```python
from build123d import *

# Parameters (mm, degrees)
BOSS_EXTRUDE1_DEPTH = 10
CUT_EXTRUDE1_DEPTH  = 7
CHAMFER2_SIZE       = 1
CHAMFER3_SIZE       = 1
SKETCH3_R           = 2.5
CUT_EXTRUDE2_DEPTH  = 10
SHELL2_START        = -7
SHELL2_DEPTH        = 14
CHAMFER4_SIZE       = 1


# Read off the part's stored shape, not the designer's step: Shell2
with BuildPart() as part:
    # Sketch1 → Boss-Extrude1 (new, symmetric)
    with BuildSketch(Plane.XY):
        with BuildLine():
            Line((-12.5, 10), (12.5, 10))
            ThreePointArc((12.5, 10), (22.5, 0), (12.5, -10))
            Line((12.5, -10), (-12.5, -10))
            ThreePointArc((-12.5, -10), (-22.5, 0), (-12.5, 10))
        make_face()
    extrude(amount=BOSS_EXTRUDE1_DEPTH, both=True)

    # Sketch2 → Cut-Extrude1 (cut, symmetric)
    with BuildSketch(Plane.XY):
        with BuildLine():
            Line((-12.5, 10), (-2.5, 10))
            Line((-2.5, 10), (-2.5, -10))
            Line((-2.5, -10), (-12.5, -10))
            ThreePointArc((-12.5, -10), (-22.5, 0), (-12.5, 10))
        make_face()
    extrude(amount=CUT_EXTRUDE1_DEPTH, both=True, mode=Mode.SUBTRACT)

    # Chamfer2
    chamfer2_edges = [part.edges().sort_by_distance(p)[0] for p in [
        (-22.5, 0, -7),
        (-7.5, 10, -7),
        (-7.5, -10, -7),
        (-22.5, 0, 7),
        (-7.5, -10, 7),
        (-7.5, 10, 7),
    ]]
    chamfer(chamfer2_edges, length=CHAMFER2_SIZE)

    # Chamfer3
    chamfer3_edges = [part.edges().sort_by_distance(p)[0] for p in [
        (22.5, 0, 10),
        (0, 10, 10),
        (-22.5, 0, 10),
        (0, 10, -10),
        (22.5, 0, -10),
        (0, -10, -10),
        (-22.5, 0, -10),
        (0, -10, 10),
    ]]
    chamfer(chamfer3_edges, length=CHAMFER3_SIZE)

    # Sketch3 → Cut-Extrude2 (cut, symmetric)
    with BuildSketch(Plane.XY):
        with Locations((-12.5, 0)):
            Circle(SKETCH3_R)
    extrude(amount=CUT_EXTRUDE2_DEPTH, both=True, mode=Mode.SUBTRACT)

    # Shell2 outline → Shell2 (cut)
    with BuildSketch(Plane.XY.offset(SHELL2_START)):
        with BuildLine():
            Line((12.5, 7), (-2.5, 7))
            Line((-2.5, 7), (-2.5, -7))
            Line((-2.5, -7), (12.5, -7))
            ThreePointArc((12.5, -7), (19.5, 0), (12.5, 7))
        make_face()
    extrude(amount=SHELL2_DEPTH, mode=Mode.SUBTRACT)

    # Chamfer4
    chamfer4_edges = [part.edges().sort_by_distance(p)[0] for p in [
        (-2.5, -10, 0),
        (-2.5, 10, 0),
    ]]
    chamfer(chamfer4_edges, length=CHAMFER4_SIZE)


solid = part.part
```
Geometry check sheet. Reference: the model listing, model coordinates, mm. A direction names the side the tool comes from. Coordinates: 2 decimals unless noted, no trailing zeros. Write each loop counter-clockwise with the first axis right and the second up, starting at its lowest first coordinate (ties: lowest second). Pieces come first, ordered by that corner, then holes. Notation, with made-up numbers: M 57.5,9.5 L 114.5,9.5 A3 ccw 114.5,14.5 Z; hole C -17.75,-37.75 d7. An arc over 180 degrees is marked long. Use one line per item in the form item = value. Start each with the question number.
1) Release check for a two-part mould opening along Z. For faces 1 (the flat face through (5, 10, 0)), 2 (the cylindrical face through (19.5, -0.15, -0.1)), 3 (the flat face through (0.2, -9.5, 9.5)) record: pulls with the +Z half, pulls with the -Z half, needs draft (parallel to the pull), parting line crosses it, or undercut.
2) Section check A-A on x = -4.5. Enter the section's corners in (y, z).
3) Section check B-B on z = -7.5. Enter the section's corners in (x, y).
4) Section check C-C on y = 0. Enter the section's corners in (x, z), and give its area (3 significant figures).
5) Go/stop test with flat-tipped pins: pin 1 Ø1.5 at (x, z) = (17.5, -6.5) entering from -Y; pin 2 Ø1.6 at (y, z) = (-8.5, -3.5) entering from -X; pin 3 Ø6 at (x, y) = (-12.5, 0) entering from +Z; pin 4 Ø8 at (y, z) = (-6.5, -4.5) entering from -X. Record where each tip stops, or that it passes through.
6) Section check D-D on x = 12. Enter the section's corners in (y, z).
7) Thickness scan on probe 1 along Z at (x, y) = (17.5, -1.25); probe 2 along Y at (x, z) = (-12.5, 8.55); probe 3 along Y at (x, z) = (-12.5, 7.75). Record the ranges inside material, lowest first. Write a range as from..to.
8) Set-up check for faces 4 (the cylindrical face through (22.5, 0.2, 0.1)), 5 (the conical face through (-21.7, -0.2, -7.2)): record each of +Z, -Z, +X, -X, +Y, -Y from which the full face is reachable in a straight line by a thin tool's end or side.
Responses:
q1.face_1 = needs draft
q1.face_2 = undercut
q1.face_3 = pulls with the +Z half
q2.outline = M -10,-9 L -9,-10 L 9,-10 L 10,-9 L 10,-8 L 9,-7 L -9,-7 L -10,-8 Z; M -10,8 L -9,7 L 9,7 L 10,8 L 10,9 L 9,10 L -9,10 L -10,9 Z
q3.outline = M -12.5,-9.5 L -2,-9.5 L -1.5,-10 L 12.5,-10 A10 ccw 12.5,10 L -1.5,10 L -2,9.5 L -12.5,9.5 A9.5 ccw Z; hole C -12.5,0 d5
q4.outline = M -22.5,-9 L -21.5,-10 L -15,-10 L -15,-7 L -21.5,-7 L -22.5,-8 Z; M -22.5,8 L -21.5,7 L -15,7 L -15,10 L -21.5,10 L -22.5,9 Z; M -10,-10 L 21.5,-10 L 22.5,-9 L 22.5,9 L 21.5,10 L -10,10 L -10,7 L 19.5,7 L 19.5,-7 L -10,-7 Z
q4.area = 279 mm2
q5.pin_1 = -9.05
q5.pin_2 = -2.5
q5.pin_3 = 10
q5.pin_4 = -21.4
q6.outline = M -10,-9 L -9,-10 L 9,-10 L 10,-9 L 10,9 L 9,10 L -9,10 L -10,9 Z; hole M -7,-7 L 7,-7 L 7,7 L -7,7 Z
q7.probe_1 = -10..-7, 7..10
q7.probe_2 = -10..-2.5, 2.5..10
q7.probe_3 = -9.75..-2.5, 2.5..9.75
q8.face_4 = +Z, -Z, +X
q8.face_5 = -X
